The listing builds one solid part. Answer for the finished solid, in the listing's coordinates (mm). A direction names the side the tool comes from. Coordinates: 2 decimals unless noted, no trailing zeros. Loops run counter-clockwise (first coordinate to the right, second up) from the corner with the lowest first, then second, coordinate; pieces in that order, holes last. Notation, with made-up numbers: (16.25, 12) - (73.25, 12) arc R28 ccw to (73.25, 37) - close; hole circle Ø1 at (69.25, -31.5). An arc over 180 degrees is marked (long way). Use one line per item in the form item = value. Start each with the question number.
```python
from build123d import *

# Parameters (mm, degrees)
BOSS_EXTRUDE5_DEPTH   = 7.62
BODY_MOVE_COPY3_ANGLE = 180
BOSS_EXTRUDE7_START   = -25.4
SKETCH7_R             = 9
BOSS_EXTRUDE7_DEPTH   = 146.05
LPATTERN1_COUNT       = 3
LPATTERN1_PITCH       = 146.05
BODY_MOVE_COPY4_ANGLE = 120
BODY_MOVE_COPY5_ANGLE = 120


with BuildPart() as part:
    # Sketch6 → Boss-Extrude5 (new body)
    with BuildSketch(Plane(origin=(0, 0, 0), x_dir=(-1, 0, 0), z_dir=(0, 1, 0))):
        with BuildLine():
            Line((-5.499261314, 15.875), (-10.998522628, 6.35))
            ThreePointArc((-10.998522628, 6.35), (0, -12.7), (10.998522628, 6.35))
            Line((10.998522628, 6.35), (5.499261314, 15.875))
            ThreePointArc((5.499261314, 15.875), (0, 19.05), (-5.499261314, 15.875))
        make_face()
    extrude(amount=BOSS_EXTRUDE5_DEPTH)


with BuildPart() as body_2:
    # Body-Move_Copy2: copy of part
    add(part.part.moved(Location((0, 60.9, 0))))


with BuildPart() as body_2_1:
    # Body-Move_Copy3: moved
    add(body_2.part.rotate(Axis((0, 0, 0), (0, 1, 0)), BODY_MOVE_COPY3_ANGLE))


with BuildPart() as part_1:
    add(part.part)

    add(body_2_1.part)  # Boss-Extrude7 merges body 2
    # Sketch7 → Boss-Extrude7 (add)
    with BuildSketch(Plane(origin=(0, 7.62, 0), x_dir=(-1, 0, 0), z_dir=(0, 1, 0)).offset(BOSS_EXTRUDE7_START)):
        with Locations(Location((0, 0, 0), (0, 0, 90))):
            Circle(SKETCH7_R)
    extrude(amount=BOSS_EXTRUDE7_DEPTH)


with BuildPart() as lpattern1_1:
    # LPattern1: pattern copy
    add(part_1.part.moved(Location(Vector(0, 1, 0) * (1 * LPATTERN1_PITCH))))


with BuildPart() as lpattern1_2:
    # LPattern1: pattern copy
    add(part_1.part.moved(Location(Vector(0, 1, 0) * (2 * LPATTERN1_PITCH))))


with BuildPart() as lpattern1_1_1:
    # Body-Move_Copy4: moved
    add(lpattern1_1.part.rotate(Axis((0, 0, 0), (0, -1, 0)), BODY_MOVE_COPY4_ANGLE))


with BuildPart() as lpattern1_2_1:
    # Body-Move_Copy5: moved
    add(lpattern1_2.part.rotate(Axis((0, 0, 0), (0, 1, 0)), BODY_MOVE_COPY5_ANGLE))

    # Combine1: union part, LPattern1_1
    add(part_1.part)
    add(lpattern1_1_1.part)


solid = lpattern1_2_1.part
```
(1) Determine the mould class of faces 5 (the face through (13.8, 210.7, -1.5)), 6 (the face through (0, -17.78, 0)), 7 (the face through (-10.808, 210.707, -6.67)) for opening direction Y: +Y half, -Y half, draft (parallel to the pull), parting line (faces both ways), or undercut.
(2) Find the intervals of material crossed by probe 1 along Y at (x, z) = (-11.5, -1); probe 2 along Y at (x, z) = (13.5, 1); probe 3 along Z at (x, y) = (1, 210), in increasing order. Write a range as from..to.
(3) Each of these flat-tipped pins is pushed along its axis until it touches: pin 1 Ø8 at (x, y) = (-11.5, 85) entering from +Z; pin 2 Ø10 at (x, y) = (6, 271.5) entering from +Z; pin 3 Ø2 at (x, z) = (11, -2) entering from +Y. Where does it stop, or does it pass through?
(4) A cutting plane is placed at A-A (y = 18.5). Determine the outline of the cut face in (x, z).
(5) For faces 1 (the face through (6.083, 390.077, -6.633)), 2 (the face through (13.71, 295.86, 1.65)), 3 (the face through (6, 0, 7)), 4 (the face through (-6, 68.52, -7)), determine the directions among +Z, -Z, +X, -X, +Y, -Y from which every point of the face is accessible in a straight line to the end or side of a thin tool.
Evaluation:
q1.face_5 = draft
q1.face_6 = -Y half
q1.face_7 = undercut
q2.probe_1 = 0..7.62, 60.9..68.52, 146.05..153.67, 206.95..214.57, 292.1..299.72, 353..360.62
q2.probe_2 = 206.95..214.57, 292.1..299.72
q2.probe_3 = -12.66..12.7
q3.pin_1 = 4.97
q3.pin_2 = 8.94
q3.pin_3 = 360.62
q4.outline = circle Ø18 at (0, 0)
q5.face_1 = +Y
q5.face_2 = +Z, +X, +Y
q5.face_3 = -Y
q5.face_4 = none
